from build123d import *

# Parameters (mm, degrees)
BOSS_EXTRUDE1_DEPTH      = 5.05
BOSS_EXTRUDE1_DEPTH_BACK = 5.05
FILLET1_R                = 5
SKETCH2_R                = 2.5
CUT_EXTRUDE1_DEPTH       = 19
FILLET2_R                = 2
CUT_EXTRUDE2_DEPTH       = 46.959928198
CUT_EXTRUDE2_DEPTH_BACK  = 46.959928198
SKETCH3_R                = 2.5


with BuildPart() as part:
    # Sketch1 → Boss-Extrude1 (new, two sides: drawn at the far end of the back side and taken through both)
    with BuildSketch(Plane.XY.offset(-BOSS_EXTRUDE1_DEPTH_BACK)):
        Polygon((-31.5, 16.75), (-31.5, -8.75), (12.160254038, -8.75), (16.160254038, -4.75), (23.160254038, -4.75), (26.903805922, -3.340808995), (31.5, 1.255385083), (31.5, 16.75), (42.5, 16.75), (42.5, 4.75), (33.884592717, -7.529037314), (20.808895905, -16.75), (-33.839745962, -16.75), (-42.5, -1.75), (-42.5, 16.75), align=None)
    extrude(amount=BOSS_EXTRUDE1_DEPTH + BOSS_EXTRUDE1_DEPTH_BACK)

    # Fillet1
    fillet1_edges = [part.edges().sort_by_distance(p)[0] for p in [
        (-31.5, -8.75, 0),
        (12.160254038, -8.75, 0),
        (16.160254038, -4.75, 0),
        (23.160254038, -4.75, 0),
        (26.903805922, -3.340808995, 0),
        (31.5, 1.255385083, 0),
        (33.884592717, -7.529037314, 0),
        (20.808895905, -16.75, 0),
        (-33.839745962, -16.75, 0),
        (-42.5, -1.75, 0),
    ]]
    fillet(fillet1_edges, radius=FILLET1_R)

    # Sketch2 → Cut-Extrude1 (cut)
    with BuildSketch(Plane(origin=(0, 16.75, 0), x_dir=(1, 0, 0), z_dir=(0, 1, 0))):
        with Locations(Location((-37, 0, 0), (0, 0, 270))):
            Circle(SKETCH2_R)
        with Locations(Location((37, 0, 0), (0, 0, 270))):
            Circle(SKETCH2_R)
    extrude(amount=-CUT_EXTRUDE1_DEPTH, mode=Mode.SUBTRACT)

    # Fillet2
    fillet2_edges = [part.edges().sort_by_distance(p)[0] for p in [
        (-31.5, 16.75, 0),
        (31.5, 16.75, 0),
        (42.5, 16.75, 0),
        (-42.5, 16.75, 0),
    ]]
    fillet(fillet2_edges, radius=FILLET2_R)

    # Sketch3 → Cut-Extrude2 (cut, two sides: drawn at the far end of the back side and taken through both)
    with BuildSketch(Plane.XY.offset(-CUT_EXTRUDE2_DEPTH_BACK)):
        with Locations((-32, -11.25)):
            Circle(SKETCH3_R)
        with Locations((18.5, -11.25)):
            Circle(SKETCH3_R)
    extrude(amount=CUT_EXTRUDE2_DEPTH + CUT_EXTRUDE2_DEPTH_BACK, mode=Mode.SUBTRACT)


solid = part.part
Work out the finished part from the listing and answer in its coordinate system (mm). A direction names the side the tool comes from. Give positions to 0.01 mm unless a question says otherwise; leave off trailing zeros. Order: outer loops, then holes, each group sorted by start corner. A loop starts at its lowest first (then second) coordinate and runs counter-clockwise, first axis right, second up. Notation, with made-up numbers: M 18,-18 L 59,-18 A14 ccw 59,2 Z; hole C -10.75,16 d6. An arc over 180 degrees is marked long. Return JSON: item names as keys, results as strings.
Q1. Find section B-B, the plane z = 3.25. State how many separate pieces and enclosed holes the cut face has, and give its area (3 significant figures).
Answer below:
{"separate pieces": "1", "enclosed holes": "2", "area": "1,030 mm^2"}
Q2. Find section D-D, the plane x = -20. Write down the section's boundary in (y, z).
Answer below:
{"outline": "M -16.75,-5.05 L -8.75,-5.05 L -8.75,5.05 L -16.75,5.05 Z"}
Q3. The mould has two halves that part along X. Classify faces 4 (the face through (28.835, -1.41, -0.071)), 5 (the face through (20.76, -16.51, 0.07)), 6 (the face through (24.94, -4.08, -0.07)), 7 (the face through (0, -11, 5.05)): pulls with the +X half, pulls with the -X half, needs draft (parallel to the pull), parting line crosses it, or undercut.
Answer below:
{"face 4": "undercut", "face 5": "pulls with the +X half", "face 6": "undercut", "face 7": "needs draft"}
Q4. Find the intervals of material crossed by line 1 along X through (y, z) = (8.25, 0); line 2 along Y through (x, z) = (18.5, 1.5); line 3 along X through (y, z) = (-11.25, -2.5), in increasing order. Write a range as [from, to].
Answer below:
{"line 1": "x = [-42.5, -39.5], [-34.5, -31.5], [31.5, 34.5], [39.5, 42.5]", "line 2": "y = [-16.75, -13.75], [-8.75, -4.75]", "line 3": "x = [-37.02, -34.5], [-29.5, 16], [21, 28.61]"}
Q5. Each of these flat-tipped pins is pushed along its axis until it touches: pin 1 (2 mm diameter, centred on y = -10.5, z = 0.5, fed in from +X); pin 2 (3 mm diameter, centred on x = -7, z = -2, fed in from +Y); pin 3 (4.5 mm diameter, centred on x = 18.5, y = -11.25, fed in from -Z); pin 4 (3 mm diameter, centred on x = 15, z = 3, fed in from +Y). Where does it stop, or does it pass through?
Answer below:
{"pin 1": "stops at x = 31.09", "pin 2": "stops at y = -8.75", "pin 3": "passes through", "pin 4": "stops at y = -5.06"}
Q6. Find section C-C, the plane y = -10. Write down the section's boundary in (x, z).
Answer below:
{"outline": "M -37.74,-5.05 L -34.17,-5.05 L -34.17,5.05 L -37.74,5.05 Z; M -29.83,-5.05 L 16.33,-5.05 L 16.33,5.05 L -29.83,5.05 Z; M 20.67,-5.05 L 30.38,-5.05 L 30.38,5.05 L 20.67,5.05 Z"}
Q7. Find section A-A, the plane y = 9. Write down the section's boundary in (x, z), and give its area (3 significant figures).
Answer below:
{"outline": "M -42.5,-5.05 L -31.5,-5.05 L -31.5,5.05 L -42.5,5.05 Z; M 31.5,-5.05 L 42.5,-5.05 L 42.5,5.05 L 31.5,5.05 Z; hole C -37,0 d5; hole C 37,0 d5", "area": "183 mm^2"}
Q8. Which of the six approach directions +Z, -Z, +X, -X, +Y, -Y give full straight-line access (tool end or side, diameter ignored) to faces 1 (the face through (-37, -2.25, 0)), 2 (the face through (39.4, 0.33, -1.19)), 3 (the face through (32.07, 16.15, 0.07))?
Answer below:
{"face 1": "+Y", "face 2": "+Z, -Z, +X, -Y", "face 3": "+Z, -Z, +Y"}
